Check sheet for the modelled part. Datum: model origin and axes. Units: mm. A direction names the side the tool comes from. Give positions to 0.01 mm unless a question says otherwise; leave off trailing zeros. Order: outer loops, then holes, each group sorted by start corner. A loop starts at its lowest first (then second) coordinate and runs counter-clockwise, first axis right, second up. Notation, with made-up numbers: (12.5, -9) - (52.5, -9) arc R9 ccw to (52.5, -4) - close; hole circle Ø8 at (82.25, 44). An arc over 180 degrees is marked (long way). Answer in a Markdown table with one row per item.
from build123d import *

# Parameters (mm, degrees)
ESQUISSE4_R             = 22.5
ESQUISSE4_R_2           = 10
BOSS_EXTRU_1_DEPTH      = 1
ESQUISSE5_R             = 11.5
BOSS_EXTRU_2_DEPTH      = 3
ENL_V_MAT_EXTRU_1_REACH = 6
ESQUISSE6_R             = 10


with BuildPart() as part:
    # Esquisse4 → Boss.-Extru.1 (new body)
    with BuildSketch(Plane(origin=(0, 0, 0), x_dir=(1, 0, 0), z_dir=(0, 1, 0))):
        with Locations(Location((0, 0, 0), (0, 0, 270))):  # turned: the seam where the file's is
            Circle(ESQUISSE4_R)
        with Locations(Location((0, 0, 0), (0, 0, 270))):  # turned: the seam where the file's is
            Circle(ESQUISSE4_R_2, mode=Mode.SUBTRACT)
    extrude(amount=BOSS_EXTRU_1_DEPTH)

    # Esquisse5 → Boss.-Extru.2 (add)
    with BuildSketch(Plane(origin=(0, 1, 0), x_dir=(1, 0, 0), z_dir=(0, 1, 0))):
        with Locations(Location((0, 0, 0), (0, 0, 270))):  # turned: the seam where the file's is
            Circle(ESQUISSE5_R)
    extrude(amount=BOSS_EXTRU_2_DEPTH)

    # Esquisse6 → Enlèv. mat.-Extru.1 (cut, up to next)
    with BuildSketch(Plane(origin=(0, 4, 0), x_dir=(1, 0, 0), z_dir=(0, 1, 0)), mode=Mode.PRIVATE) as enl_v_mat_extru_1_sk1:
        with Locations(Location((0, 0, 0), (0, 0, 270))):  # turned: the seam where the file's is
            Circle(ESQUISSE6_R)
    enl_v_mat_extru_1_tool1 = extrude(enl_v_mat_extru_1_sk1.sketch, amount=-ENL_V_MAT_EXTRU_1_REACH, mode=Mode.PRIVATE) & part.part
    add(enl_v_mat_extru_1_tool1.solids().sort_by_distance((0, 4, 0))[0], mode=Mode.SUBTRACT)


solid = part.part
(1) Cross-section at A-A, the plane z = 0. Record the cut outline in (x, y), then the cut area to 3 significant figures.
Geometry says:
| item | result |
|---|---|
| outline | (-22.5, 0) - (-10, 0) - (-10, 4) - (-11.5, 4) - (-11.5, 1) - (-22.5, 1) - close; (10, 0) - (22.5, 0) - (22.5, 1) - (11.5, 1) - (11.5, 4) - (10, 4) - close |
| area | 34.0 mm² |
(2) Gauge pin test, flat end, axial feed: P1, Ø2, axis at x = 14.5, y = 1.5, coming from the +Z side. Record the tip position at first contact, or that the pin passes through.
Geometry says:
| item | result |
|---|---|
| P1 | z = 17.9 |
(3) Thickness scan on L1, parallel to X at y = 1.1, z = 0; L2, parallel to Y at x = 7.5, z = -13; L3, parallel to X at y = 3.45, z = -1. Record the ranges inside material, lowest first.
Geometry says:
| item | result |
|---|---|
| L1 | -11.5 to -10, 10 to 11.5 |
| L2 | 0 to 1 |
| L3 | -11.46 to -9.95, 9.95 to 11.46 |
(4) Cross-section at C-C, the plane y = 3.25. Record the cut outline in (x, z), then the cut area to 3 significant figures.
Geometry says:
| item | result |
|---|---|
| outline | circle Ø23 at (0, 0); hole circle Ø20 at (0, 0) |
| area | 101 mm² |
(5) Cross-section at B-B, the plane x = 0. Record the cut outline in (y, z), then the cut area to 3 significant figures.
Geometry says:
| item | result |
|---|---|
| outline | (0, -22.5) - (1, -22.5) - (1, -11.5) - (4, -11.5) - (4, -10) - (0, -10) - close; (0, 10) - (4, 10) - (4, 11.5) - (1, 11.5) - (1, 22.5) - (0, 22.5) - close |
| area | 34.0 mm² |
(6) Cross-section at D-D, the plane x = 16. Record the cut outline in (y, z).
Geometry says:
| item | result |
|---|---|
| outline | (0, -15.82) - (1, -15.82) - (1, 15.82) - (0, 15.82) - close |
(7) Access from +Z, -Z, +X, -X, +Y, -Y to the whole of each face (thin tool, end or side, straight path). Record for faces 1 (the flat face through (-5, 0, 10)), 2 (the cylindrical face through (9.7, 2.48, 6.18)).
Geometry says:
| item | result |
|---|---|
| face 1 | +Z, -Z, +X, -X, -Y |
| face 2 | +Y |
(8) Mould release check, pull along Z, two halves, no side actions. Record for faces 3 (the cylindrical face through (-9.76, 2.03, -2.17)), 4 (the cylindrical face through (-8.618, 0.493, 20.784)), 5 (the flat face through (5, 4, -9)): pulls with the +Z half, pulls with the -Z half, needs draft (parallel to the pull), parting line crosses it, or undercut.
Geometry says:
| item | result |
|---|---|
| face 3 | undercut |
| face 4 | parting line crosses it |
| face 5 | needs draft |
